from build123d import *

# Parameters (mm, degrees)
BOSS_EXTRUDE1_START     = 40
BOSS_EXTRUDE1_DEPTH     = 3
BOSS_EXTRUDE2_DEPTH     = 3
CUT_EXTRUDE1_DEPTH      = 79.654704246
CUT_EXTRUDE1_DEPTH_BACK = 79.654704246
SKETCH2_R               = 1.5
SKETCH3_W               = 46
SKETCH3_H               = 20
BOSS_EXTRUDE4_DEPTH     = 3


with BuildPart() as part:
    # Sketch1 → Boss-Extrude1 (new body)
    with BuildSketch(Plane.XY.offset(BOSS_EXTRUDE1_START)):
        with BuildLine():
            Line((-10, 62.75), (10, 62.75))
            ThreePointArc((10, 62.75), (17.071067812, 59.821067812), (20, 52.75))
            Line((20, 52.75), (20, -52.75))
            ThreePointArc((20, -52.75), (17.071067812, -59.821067812), (10, -62.75))
            Line((10, -62.75), (-10, -62.75))
            ThreePointArc((-10, -62.75), (-17.071067812, -59.821067812), (-20, -52.75))
            Line((-20, -52.75), (-20, 52.75))
            ThreePointArc((-20, 52.75), (-17.071067812, 59.821067812), (-10, 62.75))
        make_face()
    extrude(amount=BOSS_EXTRUDE1_DEPTH)


with BuildPart() as body_2:
    # Sketch1_3 → Boss-Extrude2 (new body)
    with BuildSketch(Plane.XY):
        with BuildLine():
            Line((-10, 62.75), (10, 62.75))
            ThreePointArc((10, 62.75), (17.071067812, 59.821067812), (20, 52.75))
            Line((20, 52.75), (20, -52.75))
            ThreePointArc((20, -52.75), (17.071067812, -59.821067812), (10, -62.75))
            Line((10, -62.75), (-10, -62.75))
            ThreePointArc((-10, -62.75), (-17.071067812, -59.821067812), (-20, -52.75))
            Line((-20, -52.75), (-20, 52.75))
            ThreePointArc((-20, 52.75), (-17.071067812, 59.821067812), (-10, 62.75))
        make_face()
    extrude(amount=-BOSS_EXTRUDE2_DEPTH)


with BuildPart() as cut_extrude1_tool:
    # Sketch2 → Cut-Extrude1 (new, two sides: drawn at the far end of the back side and taken through both)
    with BuildSketch(Plane.XY.offset(-CUT_EXTRUDE1_DEPTH_BACK)):
        with Locations((0, 57.75)):
            Circle(SKETCH2_R)
        with Locations(Location((0, -57.75, 0), (0, 0, 180))):
            Circle(SKETCH2_R)
    extrude(amount=CUT_EXTRUDE1_DEPTH + CUT_EXTRUDE1_DEPTH_BACK)


with BuildPart() as part_1:
    add(part.part)

    # Cut-Extrude1: cut by cut_extrude1_tool
    add(cut_extrude1_tool.part, mode=Mode.SUBTRACT)



with BuildPart() as body_2_1:
    add(body_2.part)

    # Cut-Extrude1: cut by cut_extrude1_tool
    add(cut_extrude1_tool.part, mode=Mode.SUBTRACT)


with BuildPart() as part_2:
    add(part_1.part)

    add(body_2_1.part)  # Boss-Extrude4 merges body 2
    # Sketch3 → Boss-Extrude4 (add)
    with BuildSketch(Plane.ZY.offset(20)):
        with Locations((20, 37.75)):
            Rectangle(SKETCH3_W, SKETCH3_H)
        with Locations((20, -2.25)):
            Rectangle(SKETCH3_W, SKETCH3_H)
        with Locations((20, -42.25)):
            Rectangle(SKETCH3_W, SKETCH3_H)
    boss_extrude4 = extrude(amount=BOSS_EXTRUDE4_DEPTH)

    # Mirror1: Boss-Extrude4 across plane
    add(boss_extrude4.mirror(Plane(origin=(0, 0, 0), x_dir=(0, 0, 1), z_dir=(1, 0, 0))))


solid = part_2.part
Model file for the job. Use its own axes, mm. A direction names the side the tool comes from. Give positions to 0.01 mm unless a question says otherwise; leave off trailing zeros. Order: outer loops, then holes, each group sorted by start corner. A loop starts at its lowest first (then second) coordinate and runs counter-clockwise, first axis right, second up. Notation, with made-up numbers: (-15, 29) - (-1, 29) arc R32 cw to (-1, 56) - close; hole circle Ø2 at (17, 82.5). An arc over 180 degrees is marked (long way). Return JSON: item names as keys, results as strings.
1) Cut at A-A, the plane x = 0. Give the cut face in (y, z), plus the area to 3 significant figures.
Geometry says:
{"outline": "(-62.75, -3) - (-59.25, -3) - (-59.25, 0) - (-62.75, 0) - close; (-62.75, 40) - (-59.25, 40) - (-59.25, 43) - (-62.75, 43) - close; (-56.25, -3) - (56.25, -3) - (56.25, 0) - (-56.25, 0) - close; (-56.25, 40) - (56.25, 40) - (56.25, 43) - (-56.25, 43) - close; (59.25, -3) - (62.75, -3) - (62.75, 0) - (59.25, 0) - close; (59.25, 40) - (62.75, 40) - (62.75, 43) - (59.25, 43) - close", "area": "717 mm²"}
2) Flat gauge pins, fed straight in: P1, Ø0.9, axis at y = 14, z = 41.5, coming from the +X side; P2, Ø3.5, axis at x = 21, z = 17.5, coming from the -Y side; P3, Ø2.5, axis at x = -21, z = 14.5, coming from the +Y side; P4, Ø12, axis at y = 17.5, z = 19, coming from the +X side. Where does each tip first touch, or does it go through?
Geometry says:
{"P1": "x = 20", "P2": "y = -52.25", "P3": "y = 47.75", "P4": "through"}
3) Pull direction X, two halves, no side cores. Call faces 1 (the flat face through (-20, -42, 20)), 2 (the flat face through (0, -1, -3)), 3 (the cylindrical face through (17.15, -59.74, 41.48)): pulls with the +X half, pulls with the -X half, needs draft (parallel to the pull), parting line crosses it, or undercut.
Geometry says:
{"face 1": "undercut", "face 2": "needs draft", "face 3": "pulls with the +X half"}
4) Cut at B-B, the plane y = 12. Give the cut face in (x, z), plus the area to 3 significant figures.
Geometry says:
{"outline": "(-20, -3) - (20, -3) - (20, 0) - (-20, 0) - close; (-20, 40) - (20, 40) - (20, 43) - (-20, 43) - close", "area": "240 mm²"}
5) Cut at C-C, the plane x = -6.5. Give the cut face in (y, z).
Geometry says:
{"outline": "(-62.75, -3) - (62.75, -3) - (62.75, 0) - (-62.75, 0) - close; (-62.75, 40) - (62.75, 40) - (62.75, 43) - (-62.75, 43) - close"}
6) Cut at D-D, the plane z = 36.5. Give the cut face in (x, y).
Geometry says:
{"outline": "(-23, -52.25) - (-20, -52.25) - (-20, -32.25) - (-23, -32.25) - close; (-23, -12.25) - (-20, -12.25) - (-20, 7.75) - (-23, 7.75) - close; (-23, 27.75) - (-20, 27.75) - (-20, 47.75) - (-23, 47.75) - close; (20, -52.25) - (23, -52.25) - (23, -32.25) - (20, -32.25) - close; (20, -12.25) - (23, -12.25) - (23, 7.75) - (20, 7.75) - close; (20, 27.75) - (23, 27.75) - (23, 47.75) - (20, 47.75) - close"}
7) Probe line 1 (Z direction, x = 4.5, y = 11); line 2 (Y direction, x = 0, z = -1.95); line 3 (X direction, y = 41.5, z = 12). List the from-to ranges inside material, lowest first. Write a range as from..to.
Geometry says:
{"line 1": "-3..0, 40..43", "line 2": "-62.75..-59.25, -56.25..56.25, 59.25..62.75", "line 3": "-23..-20, 20..23"}
8) 3-axis set-ups, long thin cutter, end or side, ignore diameter. For faces 4 (the flat face through (21, 47.75, 20)), 5 (the flat face through (-21, 7.75, 20)), 6 (the flat face through (20, 18, 41)), 7 (the flat face through (0, 1, 40)), 8 (the flat face through (-20, 50, -1)): which of +Z, -Z, +X, -X, +Y, -Y reach the whole face in a straight line?
Geometry says:
{"face 4": "+Z, -Z, +X, +Y", "face 5": "+Z, -Z, -X", "face 6": "+Z, -Z, +X", "face 7": "+Y, -Y", "face 8": "+Z, -Z, -X, +Y"}
